Here's the drawing with two shaded views (mm, measured from the low corner). I have some questions. Round coordinates to 2 decimals unless told otherwise and drop trailing zeros. Loops run counter-clockwise (first coordinate to the right, second up) from the corner with the lowest first, then second, coordinate; pieces in that order, holes last. Notation, with made-up numbers: M 11,82 L 61,82 A24 ccw 61,93 Z; hole C 6.25,30.5 d2. An arc over 180 degrees is marked long. Answer as a JSON object with one key per item and string values.
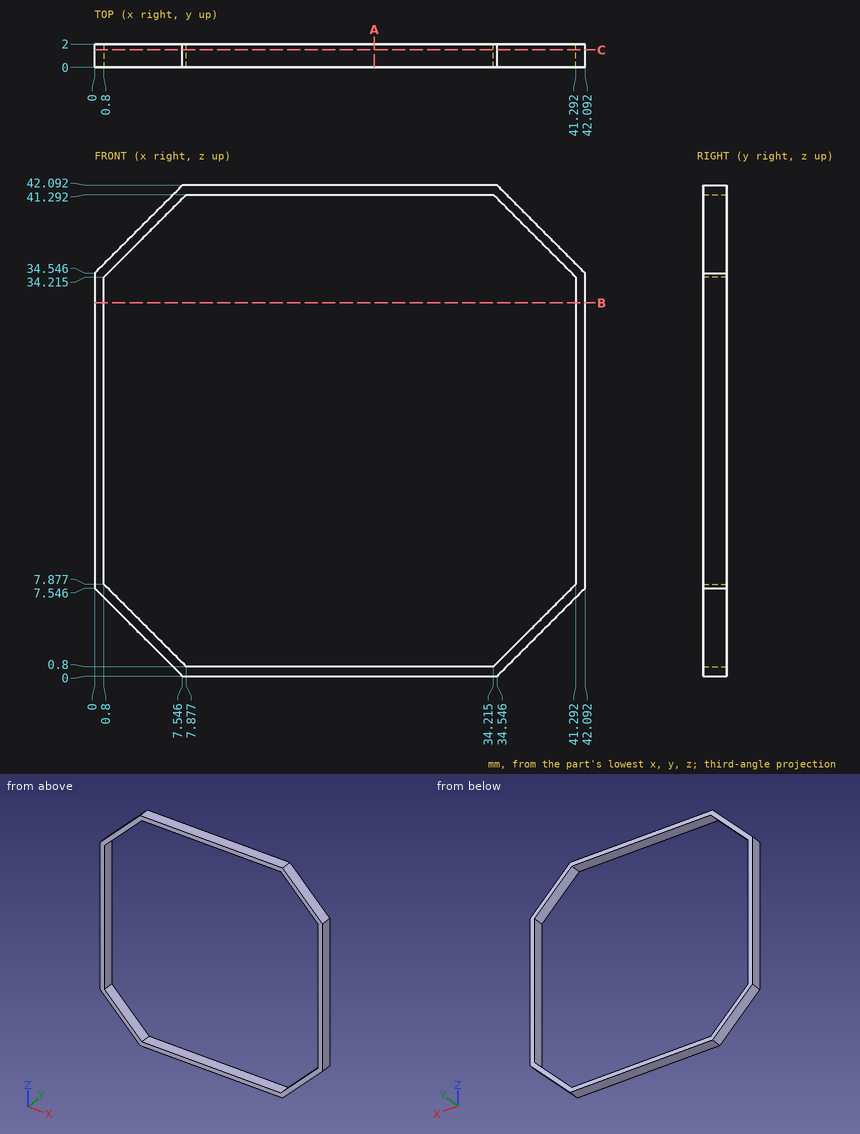
Item 1: I want a section at C-C on y = 1.5. List the corners of the cut face in (x, z) for me (1 decimal).
Solution:
{"outline": "M 0,7.5 L 7.5,0 L 34.5,0 L 42.1,7.5 L 42.1,34.5 L 34.5,42.1 L 7.5,42.1 L 0,34.5 Z; hole M 0.8,7.9 L 7.9,0.8 L 34.2,0.8 L 41.3,7.9 L 41.3,34.2 L 34.2,41.3 L 7.9,41.3 L 0.8,34.2 Z"}
Item 2: If I drill on L1, parallel to Z at x = 34, y = 0.6; L2, parallel to X at y = 1.45, z = 5.5 (1 decimal), over which ranges is the centre line in solid material (lowest first)? Write a range as from..to.
Solution:
{"L1": "z = 0..0.8, 41.29..42.09", "L2": "x = 2..3.2, 38.9..40"}
Item 3: I want a section at A-A on x = 24. List the corners of the cut face in (y, z) for me.
Solution:
{"outline": "M 0,0 L 2,0 L 2,0.8 L 0,0.8 Z; M 0,41.29 L 2,41.29 L 2,42.09 L 0,42.09 Z"}
Item 4: I want a section at B-B on z = 32. List the corners of the cut face in (x, y) for me.
Solution:
{"outline": "M 0,0 L 0.8,0 L 0.8,2 L 0,2 Z; M 41.29,0 L 42.09,0 L 42.09,2 L 41.29,2 Z"}
